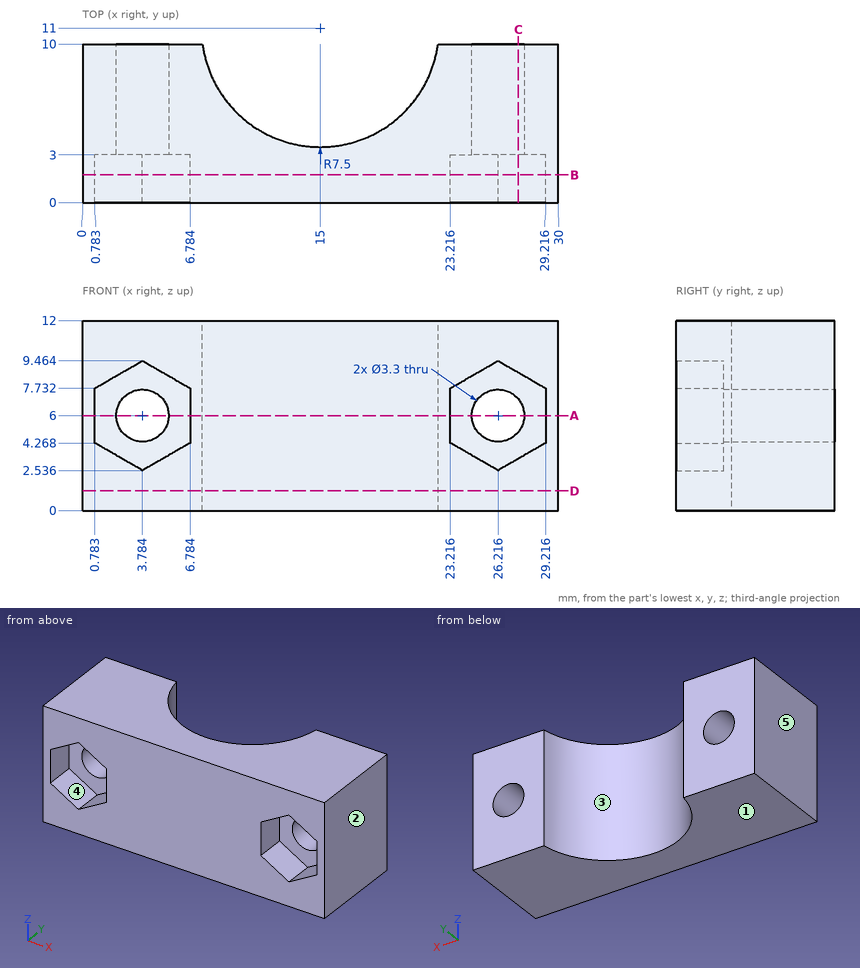
Input: dimensioned drawing with shaded views. Units: mm. Origin: part minimum x, y, z. A direction names the side the tool comes from. Give positions to 0.01 mm unless a question says otherwise; leave off trailing zeros. Order: outer loops, then holes, each group sorted by start corner. A loop starts at its lowest first (then second) coordinate and runs counter-clockwise, first axis right, second up.
(1) Section query A-A (z = 6). Return the cut outline in (x, y).
(2) Material intervals for line 1 along X through (y, z) = (2.5, 7.5); line 2 along X through (y, z) = (6, 6) (1 decimal); line 3 along X through (y, z) = (1, 9) (1 decimal), sorted ascending.
(3) Section query B-B (y = 1.75). Return the cut outline in (x, z) (1 decimal).
(4) Section query C-C (x = 27.5). Return the cut outline in (y, z).
(5) Section query D-D (z = 1.25). Return the cut outline in (x, y), plus the area to 3 significant figures.
(6) Pull-direction query (X, two-part tool) for the marked faces 1, 2 and 3; classes: +X half, -X half, draft (parallel to the pull), parting line (faces both ways), or undercut.
(7) Contact query for flat-ended pins moving along their axis: P1, Ø1.8, axis at x = 27.5, z = 6, coming from the -Y side; P2, Ø1.5, axis at x = 12.5, z = 3, coming from the +Y side; P3, Ø2, axis at x = 26.22, z = 6, coming from the -Y side; P4, Ø4, axis at x = 15, z = 7.5, coming from the +Y side. Output: stop coordinate, or through.
(8) Access query for the marked faces 4 and 5. Directions: +Z, -Z, +X, -X, +Y, -Y. A direction counts if a zero-diameter tool reaches every point of the face in a straight line with its end or side. Return the directions, or none.
Outcome:
1. outline: (0, 0) - (0.78, 0) - (0.78, 3) - (2.13, 3) - (2.13, 10) - (0, 10) - close; (5.43, 3) - (6.78, 3) - (6.78, 0) - (23.22, 0) - (23.22, 3) - (24.57, 3) - (24.57, 10) - (22.43, 10) arc R7.5 cw to (7.57, 10) - (5.43, 10) - close; (27.87, 3) - (29.22, 3) - (29.22, 0) - (30, 0) - (30, 10) - (27.87, 10) - close
2. line 1: x = 0 to 0.78, 6.78 to 23.22, 29.22 to 30
2. line 2: x = 0 to 2.1, 5.4 to 9.4, 20.6 to 24.6, 27.9 to 30
2. line 3: x = 0 to 3, 4.6 to 25.4, 27 to 30
3. outline: (0, 0) - (30, 0) - (30, 12) - (0, 12) - close; hole (0.8, 4.3) - (3.8, 2.5) - (6.8, 4.3) - (6.8, 7.7) - (3.8, 9.5) - (0.8, 7.7) - close; hole (23.2, 4.3) - (26.2, 2.5) - (29.2, 4.3) - (29.2, 7.7) - (26.2, 9.5) - (23.2, 7.7) - close
4. outline: (0, 0) - (10, 0) - (10, 4.96) - (3, 4.96) - (3, 3.28) - (0, 3.28) - close; (0, 8.72) - (3, 8.72) - (3, 7.04) - (10, 7.04) - (10, 12) - (0, 12) - close
5. outline: (0, 0) - (30, 0) - (30, 10) - (22.43, 10) arc R7.5 cw to (7.57, 10) - (0, 10) - close
5. area: 227 mm2
6. face 1: draft
6. face 2: +X half
6. face 3: undercut
7. P1: stops at y = 3
7. P2: stops at y = 4.24
7. P3: passes through
7. P4: stops at y = 3.77
8. face 4: -Y
8. face 5: +Z, -Z, -X, +Y, -Y
